The model under review builds one solid part; all positions refer to its coordinate system, in mm. A direction names the side the tool comes from. Give positions to 0.01 mm unless a question says otherwise; leave off trailing zeros. Order: outer loops, then holes, each group sorted by start corner. A loop starts at its lowest first (then second) coordinate and runs counter-clockwise, first axis right, second up. Notation, with made-up numbers: (-12.5, -38.5) - (12.5, -38.5) arc R9 ccw to (12.5, -30.5) - close; hole circle Ø7 at (22.25, -3.75). An arc over 180 degrees is marked (long way). Use CSV: the item, a comma, the result in double quotes. Start each with the question number.
```python
from build123d import *

# Parameters (mm, degrees)
BOSS_EXTRUDE1_DEPTH = 5
SKETCH5_R           = 2.6
CUT_EXTRUDE1_DEPTH  = 5
CUT_EXTRUDE2_REACH  = 55.385
SKETCH6_R           = 1.7
CUT_EXTRUDE4_REACH  = 55.385
FILLET4_R           = 1
FILLET1_R           = 5
FILLET2_R           = 2
FILLET5_R           = 1


with BuildPart() as part:
    # Sketch3 → Boss-Extrude1 (new body)
    with BuildSketch(Plane.XY):
        Polygon((20, -35), (40, -35), (40, -25), (20, -25), (20, 0), (0, 0), (0, -35), align=None)
    extrude(amount=BOSS_EXTRUDE1_DEPTH)

    # Sketch5 → Cut-Extrude1 (cut)
    with BuildSketch(Plane(origin=(0, 0, 0), x_dir=(-1, 0, 0), z_dir=(0, 0, -1))):
        with BuildLine():
            ThreePointArc((-7.4, -10), (-8.161522369, -8.161522369), (-10, -7.4))
            Line((-10, -7.4), (-10, -12.6))
            ThreePointArc((-10, -12.6), (-8.161522369, -11.838477631), (-7.4, -10))
        make_face()
        with BuildLine():
            Line((-10, -12.6), (-10, -7.4))
            ThreePointArc((-10, -7.4), (-12.6, -10), (-10, -12.6))
        make_face()
        with Locations((-10, -25)):
            Circle(SKETCH5_R)
    extrude(amount=-CUT_EXTRUDE1_DEPTH, mode=Mode.SUBTRACT)

    # Sketch6 → Cut-Extrude2 (cut, up to next)
    with BuildSketch(Plane(origin=(0, 0, 0), x_dir=(-1, 0, 0), z_dir=(0, 0, -1)), mode=Mode.PRIVATE) as cut_extrude2_sk1:
        with Locations((-27.5, -31)):
            Circle(SKETCH6_R)
    cut_extrude2_tool1 = extrude(cut_extrude2_sk1.sketch, amount=-CUT_EXTRUDE2_REACH, mode=Mode.PRIVATE) & part.part
    # Sketch6 → Cut-Extrude2 (cut, up to next)
    with BuildSketch(Plane(origin=(0, 0, 0), x_dir=(-1, 0, 0), z_dir=(0, 0, -1)), mode=Mode.PRIVATE) as cut_extrude2_sk2:
        with Locations((-33.8, -31)):
            Circle(SKETCH6_R)
    cut_extrude2_tool2 = extrude(cut_extrude2_sk2.sketch, amount=-CUT_EXTRUDE2_REACH, mode=Mode.PRIVATE) & part.part
    add(cut_extrude2_tool1.solids().sort_by_distance((27.5, -31, 0))[0], mode=Mode.SUBTRACT)
    add(cut_extrude2_tool2.solids().sort_by_distance((33.8, -31, 0))[0], mode=Mode.SUBTRACT)

    # Sketch8 → Cut-Extrude4 (cut, up to next)
    with BuildSketch(Plane(origin=(0, 0, 0), x_dir=(-1, 0, 0), z_dir=(0, 0, -1)), mode=Mode.PRIVATE) as cut_extrude4_sk1:
        Polygon((-4.5, -35), (-4.5, -33), (-5.726444717, -32), (-14.273555283, -32), (-15.5, -33), (-15.5, -35), align=None)
    cut_extrude4_tool1 = extrude(cut_extrude4_sk1.sketch, amount=-CUT_EXTRUDE4_REACH, mode=Mode.PRIVATE) & part.part
    add(cut_extrude4_tool1.solids().sort_by_distance((10, -33.545033, 0))[0], mode=Mode.SUBTRACT)

    # Fillet4
    fillet4_edges = [part.edges().sort_by_distance(p)[0] for p in [
        (5.726444717, -32, 2.5),
        (4.5, -33, 2.5),
        (15.5, -35, 2.5),
        (15.5, -33, 2.5),
        (14.273555283, -32, 2.5),
    ]]
    fillet(fillet4_edges, radius=FILLET4_R)

    # Fillet1
    # the kernel refuses this fillet: 5 mm, written as the material it adds along each edge
    with BuildSketch(Plane(origin=(20, -25, 0), x_dir=(1, 0, 0), z_dir=(0, 0, 1))) as fillet1_piece_1:
        with BuildLine():
            CenterArc((FILLET1_R, FILLET1_R), FILLET1_R, 180, 90)
            Line((0, FILLET1_R), (0, 0))
            Line((0, 0), (FILLET1_R, 0))
        make_face()
    extrude(amount=5)
    # the kernel refuses this fillet: 5 mm, written as the material it takes off along each edge
    with BuildSketch(Plane(origin=(0, -35, -12.437342964), x_dir=(0, 1, 0), z_dir=(0, 0, 1))) as fillet1_2_piece_1:
        with BuildLine():
            CenterArc((4.974937186, -5), FILLET1_R, 90, 84.260829523)
            Line((0, -4.5), (0, 0))
            Line((0, 0), (4.974937186, 0))
        make_face()
    extrude(amount=29.874685928, mode=Mode.SUBTRACT)
    with BuildSketch(Plane(origin=(0, 0, -12.5), x_dir=(1, 0, 0), z_dir=(0, 0, 1)), Plane(origin=(20, 0, -12.5), x_dir=(0, -1, 0), z_dir=(0, 0, 1))) as fillet1_2_piece_2:
        with BuildLine():
            CenterArc((FILLET1_R, -FILLET1_R), FILLET1_R, 90, 90)
            Line((0, -FILLET1_R), (0, 0))
            Line((0, 0), (FILLET1_R, 0))
        make_face()
    extrude(amount=30, mode=Mode.SUBTRACT)

    # Fillet2
    fillet2_edges = [part.edges().sort_by_distance(p)[0] for p in [
        (40, -35, 2.5),
        (40, -25, 2.5),
    ]]
    fillet(fillet2_edges, radius=FILLET2_R)

    # Fillet5
    fillet5_edges = [part.edges().sort_by_distance(p)[0] for p in [
        (4.5, -35, 2.5),
    ]]
    fillet(fillet5_edges, radius=FILLET5_R)


solid = part.part
```
1. Clearance check with flat-ended pins moving along their axes: pin 1 (4 mm diameter, centred on x = 27.5, y = -31, fed in from +Z); pin 2 (2.5 mm diameter, centred on x = 10.5, z = 1.5, fed in from -Y); pin 3 (3 mm diameter, centred on x = 34, z = 1, fed in from +Y); pin 4 (1.5 mm diameter, centred on y = -12, z = 3, fed in from +X). State where each tip first meets the part, or that it passes through.
2. Consider section A-A (z = 2.75). Give the boundary of the cut face in (x, y) (3 decimals).
3. Consider section D-D (y = -9.5). Give the boundary of the cut face in (x, z), and give its area (3 significant figures).
4. Consider section B-B (x = 33.8). Give the boundary of the cut face in (y, z).
5. To check wall thickness, follow L1, parallel to Y at x = 10, z = 2.1; L2, parallel to Y at x = 33.8, z = 2.15; L3, parallel to X at y = -30, z = 1.7. State the ranges of each line that lie inside material, in increasing order. Write a range as [from, to].
6. Consider section C-C (y = -31). Give the boundary of the cut face in (x, z), and give its area (3 significant figures).
7. Tool access review of faces 4 (the face through (20, -13, 2)), 5 (the face through (15.801, -34.715, 2.535)), 6 (the face through (16, -21, 0)): name each direction out of +Z, -Z, +X, -X, +Y, -Y from which nothing blocks a thin tool from reaching the whole face with its end or side.
8. Mouldability with a two-part tool opening along X and no side actions: class faces 1 (the face through (19, -2, 2)), 2 (the face through (4.07, -34.555, 2.535)), 3 (the face through (10, 0, 2)) as pulls with the +X half, pulls with the -X half, needs draft (parallel to the pull), parting line crosses it, or undercut.
Answers follow:
1,pin 1,"stops at z = 5"
1,pin 2,"stops at y = -32"
1,pin 3,"stops at y = -25"
1,pin 4,"stops at x = 20"
2,outline,"(0, -30.025) arc R5 ccw to (3.125, -34.66) arc R1 ccw to (4.5, -33.733) - (4.5, -33.475) arc R1 cw to (4.868, -32.7) - (5.451, -32.225) arc R1 cw to (6.082, -32) - (13.918, -32) arc R1 cw to (14.549, -32.225) - (15.132, -32.7) arc R1 cw to (15.5, -33.475) - (15.5, -34) arc R1 ccw to (16.5, -35) - (38, -35) arc R2 ccw to (40, -33) - (40, -27) arc R2 ccw to (38, -25) - (25, -25) arc R5 cw to (20, -20) - (20, -5) arc R5 ccw to (15, 0) - (5, 0) arc R5 ccw to (0, -5) - close; hole circle Ø5.2 at (10, -25); hole circle Ø5.2 at (10, -10); hole circle Ø3.4 at (27.5, -31); hole circle Ø3.4 at (33.8, -31)"
3,outline,"(0, 0) - (7.45, 0) - (7.45, 5) - (0, 5) - close; (12.55, 0) - (20, 0) - (20, 5) - (12.55, 5) - close"
3,area,"74.5 mm^2"
4,outline,"(-35, 0) - (-32.7, 0) - (-32.7, 5) - (-35, 5) - close; (-29.3, 0) - (-25, 0) - (-25, 5) - (-29.3, 5) - close"
5,L1,"y = [-32, -27.6], [-22.4, -12.6], [-7.4, 0]"
5,L2,"y = [-35, -32.7], [-29.3, -25]"
5,L3,"x = [0, 26.13], [28.87, 32.43], [35.17, 40]"
6,outline,"(0.1, 0) - (25.8, 0) - (25.8, 5) - (0.1, 5) - close; (29.2, 0) - (32.1, 0) - (32.1, 5) - (29.2, 5) - close; (35.5, 0) - (40, 0) - (40, 5) - (35.5, 5) - close"
6,area,"166 mm^2"
7,face 4,"+Z, -Z, +X, +Y"
7,face 5,"+Z, -Z, -Y"
7,face 6,"-Z, +X, -X, +Y, -Y"
8,face 1,"pulls with the +X half"
8,face 2,"undercut"
8,face 3,"needs draft"
